Check sheet for the modelled part. Datum: model origin and axes. Units: mm. A direction names the side the tool comes from. Round coordinates to 2 decimals unless told otherwise and drop trailing zeros. Order: outer loops, then holes, each group sorted by start corner. A loop starts at its lowest first (then second) coordinate and runs counter-clockwise, first axis right, second up. Notation, with made-up numbers: (46.5, 75) -> (84.5, 75) arc R29 ccw to (84.5, 106) -> close; hole circle Ø6 at (3.5, 42). An arc over 180 degrees is marked (long way). Answer in a Markdown table with one row per item.
```python
from build123d import *

# Parameters (mm, degrees)
SKETCH_1_W                  = 86
SKETCH_1_H                  = 43
EXTRUDE_1_DEPTH             = 39.5
EXTRUDE_2_DEPTH             = 5
SKETCH_3_W                  = 80.6
SKETCH_3_H                  = 40.2
CUT_EXTRUDE_1_DEPTH         = 43.6
HOLE_WIZARD_8_3_8_3_1_D     = 8.3
HOLE_WIZARD_8_3_8_3_1_DEPTH = 3.2
FILLET_1_R                  = 3
EXTRUDE_START               = -4
SKETCH_6_R                  = 4.15
EXTRUDE_3_DEPTH             = 4
EXTRUDE_4_DEPTH             = 42
FILLET_2_R                  = 2


with BuildPart() as part:
    # Эскиз1 → Бобышка-Вытянуть1 (new body)
    with BuildSketch(Plane.XY.offset(22.25)):
        with Locations((47, 0)):
            Rectangle(SKETCH_1_W, SKETCH_1_H)
    extrude(amount=-EXTRUDE_1_DEPTH)

    # Эскиз2 → Бобышка-Вытянуть2 (add)
    with BuildSketch(Plane(origin=(0, 0, -17.25), x_dir=(-1, 0, 0), z_dir=(0, 0, -1))):
        with BuildLine():
            Line((-90, -21.5), (-90, -16.5))
            ThreePointArc((-90, -16.5), (-104, 0), (-90, 16.5))
            Line((-90, 16.5), (-90, 21.5))
            Line((-90, 21.5), (-4, 21.5))
            Line((-4, 21.5), (-4, -21.5))
            Line((-4, -21.5), (-90, -21.5))
        make_face()
        with BuildLine():
            Line((-90, -12.428366172), (-90, 12.428366172))
            ThreePointArc((-90, 12.428366172), (-100, 0), (-90, -12.428366172))
        make_face(mode=Mode.SUBTRACT)
    extrude(amount=EXTRUDE_2_DEPTH)

    # Эскиз3 → Вырез-Вытянуть1 (cut)
    with BuildSketch(Plane.XY.offset(22.25)):
        with Locations((48.3, 0)):
            Rectangle(SKETCH_3_W, SKETCH_3_H)
    extrude(amount=-CUT_EXTRUDE_1_DEPTH, mode=Mode.SUBTRACT)

    # Диаметр отверстия Ø8.3 (8.3)1
    with Locations(Plane.ZY.offset(-4)):
        with Locations((0, 0)):
            Hole(HOLE_WIZARD_8_3_8_3_1_D / 2, depth=HOLE_WIZARD_8_3_8_3_1_DEPTH)

    # Скругление1
    fillet_1_edges = [part.edges().sort_by_distance(p)[0] for p in [
        (4, -21.5, 0),
        (4, 21.5, 0),
    ]]
    fillet(fillet_1_edges, radius=FILLET_1_R)

    # Эскиз6 → Бобышка-Вытянуть3 (add)
    with BuildSketch(Plane.ZY.offset(-4).offset(EXTRUDE_START)):
        Circle(SKETCH_6_R)
    extrude(amount=EXTRUDE_3_DEPTH)

    # Эскиз7 → Бобышка-Вытянуть4 (add)
    with BuildSketch(Plane(origin=(0, 0, -22.25), x_dir=(-1, 0, 0), z_dir=(0, 0, -1))):
        Polygon((-90, -1.1), (-90, 1.1), (-4, 1.1), (-4, 0), (-4, -1.1), align=None)
    extrude(amount=-EXTRUDE_4_DEPTH)

    # Скругление2
    fillet_2_edges = [part.edges().sort_by_distance(p)[0] for p in [
        (48.3, -20.1, -21.35),
        (88.6, -20.1, 0.45),
        (8, 10.6, -21.35),
        (8, -20.1, 0.45),
        (48.3, 20.1, -21.35),
        (8, 20.1, 0.45),
        (88.6, -10.6, -21.35),
        (88.6, 20.1, 0.45),
        (88.6, 10.6, -21.35),
        (8, -10.6, -21.35),
        (48.3, -1.1, -21.35),
        (48.3, 1.1, -21.35),
        (8, 1.1, -0.8),
        (88.6, 1.1, -0.8),
        (8, -1.1, -0.8),
        (88.6, -1.1, -0.8),
    ]]
    fillet(fillet_2_edges, radius=FILLET_2_R)


solid = part.part
```
(1) Tool access check on faces 1 (the flat face through (4, 0, 0)), 2 (the cylindrical face through (48.84, 19.5, -20.78)). Record the directions out of +Z, -Z, +X, -X, +Y, -Y that give a thin tool (end or side, any length) a straight path to the whole face; none if there is none.
Solutions:
| item | result |
|---|---|
| face 1 | +Z, -Z, -X, +Y, -Y |
| face 2 | +Z |
(2) Depth check by flat-ended pin: pin 1 Ø4 at (y, z) = (16, 1.5) entering from +X; pin 2 Ø1.9 at (x, y) = (48.5, 1.5) entering from +Z; pin 3 Ø7.5 at (x, y) = (35.5, 12.5) entering from +Z. Enter the tip coordinate at first touch or a pass-through.
Solutions:
| item | result |
|---|---|
| pin 1 | x = 90 |
| pin 2 | z = 19.75 |
| pin 3 | z = -21.35 |
(3) Scan lines: probe 1 along Y at (x, z) = (19, 10); probe 2 along X at (y, z) = (-11, 7); probe 3 along Y at (x, z) = (13, -20). Record each from-to range of solid material in increasing order. Write a range as from..to.
Solutions:
| item | result |
|---|---|
| probe 1 | -21.5..-20.1, -1.1..1.1, 20.1..21.5 |
| probe 2 | 4..8, 88.6..90 |
| probe 3 | -21.5..-19.99, -1.21..1.21, 19.99..21.5 |
(4) Section check D-D on y = 10. Record the boundary of the cut face in (x, z), plus the area to 3 significant figures.
Solutions:
| item | result |
|---|---|
| outline | (4, -22.25) -> (90, -22.25) -> (90, 22.25) -> (88.6, 22.25) -> (88.6, -19.35) arc R2 cw to (86.6, -21.35) -> (10, -21.35) arc R2 cw to (8, -19.35) -> (8, 22.25) -> (4, 22.25) -> close; (95.14, -22.25) -> (100.68, -22.25) -> (100.68, -17.25) -> (95.14, -17.25) -> close |
| area | 342 mm^2 |
(5) Draft check along Y on faces 3 (the cylindrical face through (104, 0, -20)), 4 (the flat face through (48, -20.1, 2)), 5 (the flat face through (102, 0, -17.25)). Enter one of: pulls with the +Y half, pulls with the -Y half, needs draft (parallel to the pull), parting line crosses it, or undercut.
Solutions:
| item | result |
|---|---|
| face 3 | parting line crosses it |
| face 4 | undercut |
| face 5 | needs draft |
(6) Section check C-C on x = 14. Record the boundary of the cut face in (y, z), plus the area to 3 significant figures.
Solutions:
| item | result |
|---|---|
| outline | (-21.5, -22.25) -> (21.5, -22.25) -> (21.5, 22.25) -> (20.1, 22.25) -> (20.1, -19.35) arc R2 cw to (18.1, -21.35) -> (3.1, -21.35) arc R2 cw to (1.1, -19.35) -> (1.1, 19.75) -> (-1.1, 19.75) -> (-1.1, -19.35) arc R2 cw to (-3.1, -21.35) -> (-18.1, -21.35) arc R2 cw to (-20.1, -19.35) -> (-20.1, 22.25) -> (-21.5, 22.25) -> close |
| area | 255 mm^2 |
(7) Section check B-B on y = -11. Record the boundary of the cut face in (x, z), plus the area to 3 significant figures.
Solutions:
| item | result |
|---|---|
| outline | (4, -22.25) -> (90, -22.25) -> (90, 22.25) -> (88.6, 22.25) -> (88.6, -19.35) arc R2 cw to (86.6, -21.35) -> (10, -21.35) arc R2 cw to (8, -19.35) -> (8, 22.25) -> (4, 22.25) -> close; (93.67, -22.25) -> (99.87, -22.25) -> (99.87, -17.25) -> (93.67, -17.25) -> close |
| area | 346 mm^2 |
(8) Section check A-A on z = -5. Record the boundary of the cut face in (x, y), plus the area to 3 significant figures.
Solutions:
| item | result |
|---|---|
| outline | (4, -18.5) arc R3 ccw to (7, -21.5) -> (90, -21.5) -> (90, 21.5) -> (7, 21.5) arc R3 ccw to (4, 18.5) -> close; hole (8, -18.1) arc R2 ccw to (10, -20.1) -> (86.6, -20.1) arc R2 ccw to (88.6, -18.1) -> (88.6, -3.1) arc R2 ccw to (86.6, -1.1) -> (10, -1.1) arc R2 ccw to (8, -3.1) -> close; hole (8, 3.1) arc R2 ccw to (10, 1.1) -> (86.6, 1.1) arc R2 ccw to (88.6, 3.1) -> (88.6, 18.1) arc R2 ccw to (86.6, 20.1) -> (10, 20.1) arc R2 ccw to (8, 18.1) -> close |
| area | 638 mm^2 |
